from build123d import *

# Parameters (mm, degrees)
BOSS_EXTRUDE1_DEPTH   = 10
F_2_0MM_DOWEL_HOLE1_D = 2
FILLET1_R             = 10
FILLET2_R             = 2.5


with BuildPart() as part:
    # Sketch1 → Boss-Extrude1 (new body)
    with BuildSketch(Plane(origin=(0, 0, 0), x_dir=(1, 0, 0), z_dir=(0, 1, 0))):
        with BuildLine():
            Line((146.108539292, 1980.364966037), (146.108539292, 1898.164966235))
            ThreePointArc((146.108539292, 1898.164966235), (204.100938953, 1758.158928457), (344.106976731, 1700.166528796))
            Line((344.106976731, 1700.166528796), (344.106976731, 1750.166528796))
            ThreePointArc((344.106976731, 1750.166528796), (239.456278012, 1793.514267516), (196.108539292, 1898.164966235))
            Line((196.108539292, 1898.164966235), (242.106976731, 1898.164966235))
            Line((242.106976731, 1898.164966235), (242.106976731, 1959.364966037))
            Line((242.106976731, 1959.364966037), (246.106976731, 1959.364966037))
            Line((246.106976731, 1959.364966037), (246.106976731, 1984.364966037))
            Line((246.106976731, 1984.364966037), (146.108539292, 1984.364966037))
            Line((146.108539292, 1984.364966037), (146.108539292, 1980.364966037))
        make_face()
    extrude(amount=-BOSS_EXTRUDE1_DEPTH)

    # Ø2.0mm Dowel Hole1 (through all)
    with Locations(Plane(origin=(0, 0, 0), x_dir=(1, 0, 0), z_dir=(0, 1, 0))):
        with Locations((175.906976731, 1981.364966037), (232.106976731, 1981.364966037), (243.106976731, 1970.364966037)):
            Hole(F_2_0MM_DOWEL_HOLE1_D / 2)

    # Fillet1
    # the kernel refuses this fillet: 10 mm, written as the material it adds along each edge
    with BuildSketch(Plane(origin=(196.108539292, 0, -1898.164966235), x_dir=(0.03625613161983894, 0, 0.9993425303267969), z_dir=(0, -1, 0))) as fillet1_piece_1:
        with BuildLine():
            CenterArc((10.369140338, -9.993425303), FILLET1_R, 87.922221298, 94.155557404)
            Line((0.375715035, -10.355986619), (0, 0))
            ThreePointArc((0, 0), (5.365850827, 0.097304484), (10.731701655, 0))
        make_face()
    extrude(amount=10)
    with BuildSketch(Plane(origin=(242.106976731, 0, -1959.364966037), x_dir=(1, 0, 0), z_dir=(0, -1, 0))) as fillet1_piece_2:
        with BuildLine():
            CenterArc((10, 8), FILLET1_R, 180, 53.130102354)
            Line((0, 8), (0, 0))
            Line((0, 0), (4, 0))
        make_face()
    extrude(amount=10)
    # the kernel refuses this fillet: 10 mm, written as the material it takes off along each edge
    with BuildSketch(Plane(origin=(146.108539292, 25, -1984.364966037), x_dir=(0, 0, 1), z_dir=(0, -1, 0)), Plane(origin=(246.106976731, 25, -1984.364966037), x_dir=(-1, 0, 0), z_dir=(0, -1, 0))) as fillet1_2_piece_1:
        with BuildLine():
            CenterArc((FILLET1_R, -FILLET1_R), FILLET1_R, 90, 90)
            Line((0, -FILLET1_R), (0, 0))
            Line((0, 0), (FILLET1_R, 0))
        make_face()
    extrude(amount=60, mode=Mode.SUBTRACT)
    with BuildSketch(Plane(origin=(242.106976731, 25, -1898.164966235), x_dir=(-1, 0, 0), z_dir=(0, -1, 0))) as fillet1_2_piece_2:
        with BuildLine():
            CenterArc((FILLET1_R, FILLET1_R), FILLET1_R, 180, 90)
            Line((0, FILLET1_R), (0, 0))
            Line((0, 0), (FILLET1_R, 0))
        make_face()
    extrude(amount=60, mode=Mode.SUBTRACT)

    # Fillet2
    fillet2_edges = [part.edges().sort_by_distance(p)[0] for p in [
        (246.106976731, -5, -1959.364966037),
    ]]
    fillet(fillet2_edges, radius=FILLET2_R)


solid = part.part
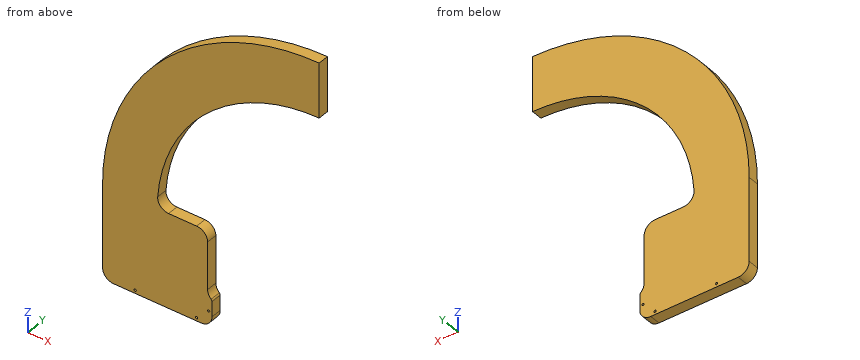
Design review of the part built by this model. Coordinates are the model's own, in mm. Give positions to 0.01 mm unless a question says otherwise; leave off trailing zeros. Loops run counter-clockwise (first coordinate to the right, second up) from the corner with the lowest first, then second, coordinate; pieces in that order, holes last. Notation, with made-up numbers: (-1.75, 1) -> (57.25, 1) arc R18 ccw to (57.25, 24) -> close; hole circle Ø6 at (-11.5, -27). An arc over 180 degrees is marked (long way). One line per question, with ' | ' between items. Start each with the question number.
(1) We need section A-A (x = 227). State the section outline as (y, z) points, and give its area (3 significant figures).
(2) Insertion check: P1, Ø1.8, axis at x = 175.91, z = -1981.36, coming from the +Y side; P2, Ø3, axis at y = -4, z = -1921, coming from the +X side; P3, Ø5, axis at y = -7, z = -1770.5, coming from the +X side; P4, Ø1.5, axis at x = 283.5, y = -6, coming from the -Z side. Each pin has a flat end and moves straight along its axis. Give the tip position at first contact, or say it passes through.
(3) We need section B-B (y = -8.5). State the section outline as (x, z) points, and give its area (3 significant figures).
(4) We need section C-C (z = -1861). State the section outline as (x, y) points, and give its area (3 significant figures).
(5) We need section D-D (x = 278). State the section outline as (y, z) points.
(6) For line 1 (X direction, y = -9, z = -1728.5); line 2 (Z direction, x = 297.5, y = -0.75); line 3 (Z direction, x = 289, y = -9), list the stretches that pass through material, from the lowest coordinate up.
The answers:
1) outline: (-10, -1984.36) -> (0, -1984.36) -> (0, -1898.16) -> (-10, -1898.16) -> close; (-10, -1807.67) -> (0, -1807.67) -> (0, -1738.51) -> (-10, -1738.51) -> close | area: 1,550 mm^2
2) P1: passes through | P2: stops at x = 242.11 | P3: stops at x = 273.68 | P4: stops at z = -1763.48
3) outline: (146.11, -1974.36) arc R10 ccw to (156.11, -1984.36) -> (236.11, -1984.36) arc R10 ccw to (246.11, -1974.36) -> (246.11, -1960.53) arc R2.5 ccw to (245.31, -1958.7) arc R10 cw to (242.11, -1951.36) -> (242.11, -1908.16) arc R10 ccw to (232.11, -1898.16) -> (206.47, -1898.16) arc R10 cw to (196.5, -1887.44) arc R148 cw to (344.11, -1750.17) -> (344.11, -1700.17) arc R198 ccw to (146.11, -1898.16) -> close; hole circle Ø2 at (175.91, -1981.36); hole circle Ø2 at (232.11, -1981.36); hole circle Ø2 at (243.11, -1970.36) | area: 21,900 mm^2
4) outline: (149.63, -10) -> (200.85, -10) -> (200.85, 0) -> (149.63, 0) -> close | area: 512 mm^2
5) outline: (-10, -1765.75) -> (0, -1765.75) -> (0, -1711.53) -> (-10, -1711.53) -> close
6) line 1: x = 242.04 to 344.11 | line 2: z = -1757.7 to -1705.73 | line 3: z = -1760.81 to -1707.99
